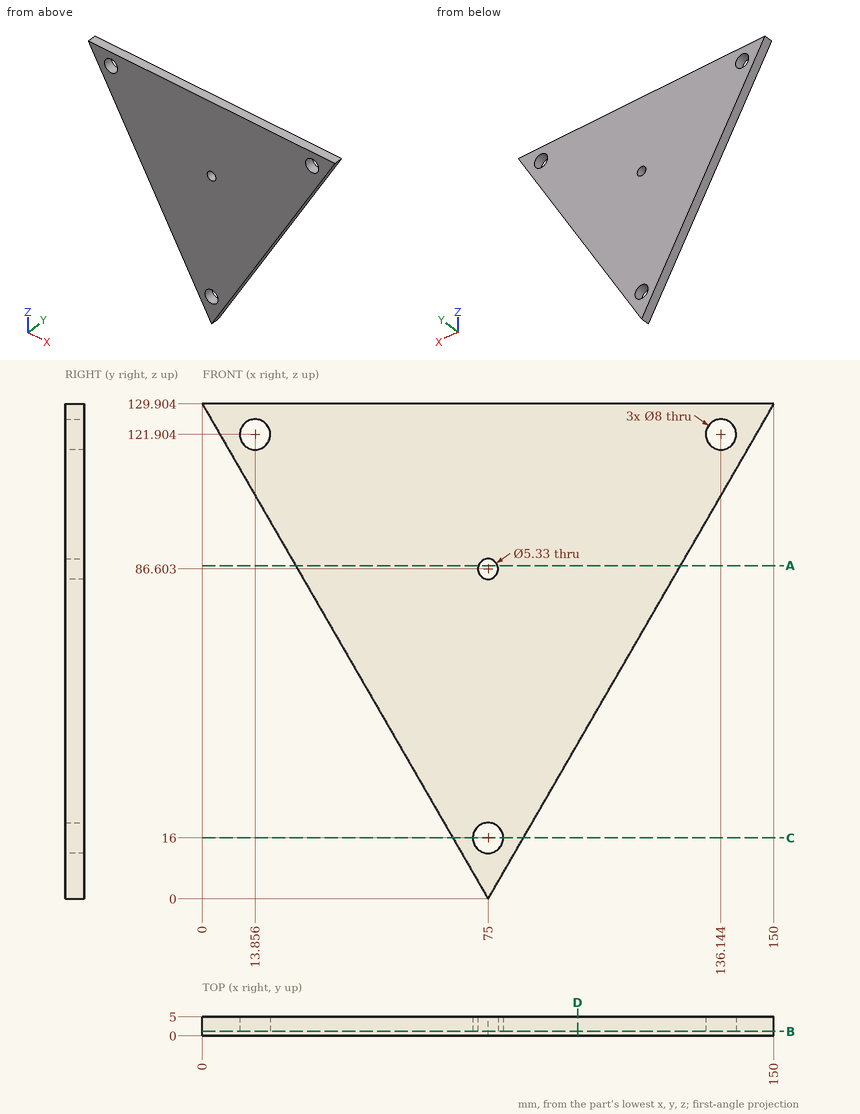
Drawing for the job (mm, zero at the part's lowest x, y, z). Give positions to 0.01 mm unless a question says otherwise; leave off trailing zeros. Loops run counter-clockwise (first coordinate to the right, second up) from the corner with the lowest first, then second, coordinate; pieces in that order, holes last.
1) Band-saw the part on A-A on z = 87.5. List the corners of the cut face in (x, y).
Values follow:
outline: (24.48, 0) - (72.49, 0) - (72.49, 5) - (24.48, 5) - close; (77.51, 0) - (125.52, 0) - (125.52, 5) - (77.51, 5) - close
2) Drop flat-ended pins along their axis: P1, Ø3, axis at y = 4, z = 113, coming from the -X side; P2, Ø2, axis at y = 3.5, z = 63, coming from the -X side. Give the stop position or say it passes through.
Values follow:
P1: stops at x = 8.89
P2: stops at x = 38.05
3) Band-saw the part on D-D on x = 98.5. List the corners of the cut face in (y, z), then the cut area to 3 significant figures.
Values follow:
outline: (0, 40.7) - (5, 40.7) - (5, 129.9) - (0, 129.9) - close
area: 446 mm2
4) Probe line 1 along Z through (x, y) = (75, 3.4) (1 decimal); line 2 along X through (y, z) = (2.7, 120) (1 decimal); line 3 along X through (y, z) = (3.7, 16). List the from-to ranges inside material, lowest first.
Values follow:
line 1: z = 0 to 12, 20 to 83.9, 89.3 to 129.9
line 2: x = 5.7 to 10.3, 17.4 to 132.6, 139.7 to 144.3
line 3: x = 65.76 to 71, 79 to 84.24
5) Band-saw the part on B-B on y = 1.2. List the corners of the cut face in (x, z) (1 decimal), then the cut area to 3 significant figures.
Values follow:
outline: (0, 129.9) - (75, 0) - (150, 129.9) - close; hole circle Ø8 at (13.9, 121.9); hole circle Ø8 at (75, 16); hole circle Ø5.3 at (75, 86.6); hole circle Ø8 at (136.1, 121.9)
area: 9,570 mm2
6) Band-saw the part on C-C on z = 16. List the corners of the cut face in (x, y).
Values follow:
outline: (65.76, 0) - (71, 0) - (71, 5) - (65.76, 5) - close; (79, 0) - (84.24, 0) - (84.24, 5) - (79, 5) - close
